from build123d import *

# Parameters (mm, degrees)
F0_R     = 20
F1_DEPTH = 80
F4_D     = 10
F4_DEPTH = 30
F4_START = 0.6350834
F4_TIP   = 3.0043030951
F5_R     = 5
F6_R     = 5


with BuildPart() as f1:
    # F0 (on Front) → F1 (new body)
    with BuildSketch(Plane.XZ):
        Circle(F0_R)
    extrude(amount=F1_DEPTH)

    # F4
    # its depths count from where the whole tool has entered the part; down to there all is cleared
    with Locations(Plane.YZ.offset(20).offset(-F4_START)):
        with Locations((-40, 0)):
            Hole(F4_D / 2, depth=F4_DEPTH)
            with Locations((0, 0, -(F4_DEPTH + F4_TIP / 2))):  # 118° drill point
                Cone(0, F4_D / 2, F4_TIP, mode=Mode.SUBTRACT)

    # F5
    f5_edges = [f1.edges().sort_by_distance(p)[0] for p in [
        (-20, 0, 0),
    ]]
    fillet(f5_edges, radius=F5_R)

    # F6
    f6_edges = [f1.edges().sort_by_distance(p)[0] for p in [
        (-20, -80, 0),
    ]]
    fillet(f6_edges, radius=F6_R)


solid = f1.part
Can you work these out from the model? Positions are in its coordinate system, mm. A direction names the side the tool comes from. Coordinates: 2 decimals unless noted, no trailing zeros. Write each loop counter-clockwise with the first axis right and the second up, starting at its lowest first coordinate (ties: lowest second). Pieces come first, ordered by that corner, then holes. Notation, with made-up numbers: (68, 72) -> (92, 72) arc R31 ccw to (92, 96) -> close; hole circle Ø10 at (74, 52). An arc over 180 degrees is marked (long way). Write each question's results on one line, items separated by ' | '. Start each with the question number.
Q1. We'd pull the mould along Y, two halves only. Please class faces 3 (the face through (0, -80, 0)), 4 (the face through (-13.12, -39.2, -0.33)), 5 (the face through (0, 0, 0)): +Y half, -Y half, draft (parallel to the pull), parting line (faces both ways), or undercut.
Q2. Imagine slicing it at B-B (y = -8). Write out the boundary of the cut face in (x, z).
Q3. If I drill on probe 1 along Y at (x, z) = (-4, 0); probe 2 along Z at (x, y) = (12, -40); probe 3 along Z at (x, y) = (9, -40), over which ranges is the centre line in solid material (lowest first)?
Q4. Imagine slicing it at A-A (x = 0). Write out the boundary of the cut face in (y, z).
Q5. I'm going to push flat-ended pins straight in: pin 1 (1 mm diameter, centred on y = -37, z = 8.5, fed in from +X); pin 2 (3 mm diameter, centred on x = -16, y = -10.5, fed in from +Z) (3 decimals); pin 3 (8 mm diameter, centred on y = -26.5, z = -7, fed in from +X); pin 4 (6 mm diameter, centred on x = 3.5, z = -3.5, fed in from +Y). Where does each tip first touch, or does it pass through?
Q6. On a 3-axis mill with a long thin cutter (end or side, diameter ignored), from which of +Z, -Z, +X, -X, +Y, -Y can I reach the whole of each face in a straight line? I mean faces 1 (the face through (-4.336, -39.51, -19.524)), 2 (the face through (4, -35, 0)). Say none if no direction works.
Taken from the geometry:
1) face 3: -Y half | face 4: undercut | face 5: +Y half
2) outline: circle Ø40 at (0, 0)
3) probe 1: y = -80 to -45, -35 to 0 | probe 2: z = -16 to -5, 5 to 16 | probe 3: z = -17.86 to -5, 5 to 17.86
4) outline: (-80, -15) arc R5 ccw to (-75, -20) -> (-5, -20) arc R5 ccw to (0, -15) -> (0, 15) arc R5 ccw to (-5, 20) -> (-75, 20) arc R5 ccw to (-80, 15) -> close; hole circle Ø10 at (-40, 0)
5) pin 1: stops at x = 18.33 | pin 2: stops at z = 13.775 | pin 3: stops at x = 19.77 | pin 4: stops at y = 0
6) face 1: +Y, -Y | face 2: +X
